```python
from build123d import *

# Parameters (mm, degrees)
F0_W     = 3.175
F0_H     = 3.175
F1_DEPTH = 6.35
F2_W     = 41.275
F2_H     = 28.575
F3_DEPTH = 6.35
F4_D     = 2.2606
F5_D     = 2.2606
F6_D     = 2.2606
F7_D     = 2.2606
F8_D     = 2.2606
F9_D     = 2.2606
F10_D    = 2.2606
F11_D    = 2.2606
F12_D    = 2.2606
F13_D    = 2.2606
F14_D    = 2.2606
F15_D    = 2.2606


with BuildPart() as f1:
    # F0 (on Top) → F1 (new body)
    with BuildSketch(Plane.XY):
        with Locations((1.5875, 1.5875)):
            Rectangle(F0_W, F0_H)
        Polygon((3.175, 3.175), (3.175, 0), (50.8, 0), (50.8, 3.175), (53.975, 3.175), (53.975, 38.1), (50.8, 38.1), (50.8, 41.275), (3.175, 41.275), (3.175, 38.1), (0, 38.1), (0, 3.175), align=None)
        with Locations((52.3875, 1.5875)):
            Rectangle(F0_W, F0_H)
        with Locations((1.5875, 39.6875)):
            Rectangle(F0_W, F0_H)
        with Locations((52.3875, 39.6875)):
            Rectangle(F0_W, F0_H)
    extrude(amount=F1_DEPTH)

    # F2 (on face) → F3 (cut, through all)
    with BuildSketch(Plane(origin=(0, 0, 0), x_dir=(1, 0, 0), z_dir=(0, 0, -1))):
        with Locations((26.9875, -20.6375)):
            Rectangle(F2_W, F2_H)
    extrude(amount=-F3_DEPTH, mode=Mode.SUBTRACT)

    # F4 (through all)
    with Locations(Plane(origin=(0, 0, 0), x_dir=(1, 0, 0), z_dir=(0, 0, -1))):
        with Locations((11.1125, -3.175)):
            Hole(F4_D / 2)

    # F5 (through all)
    with Locations(Plane(origin=(0, 0, 0), x_dir=(1, 0, 0), z_dir=(0, 0, -1))):
        with Locations((21.43125, -3.175)):
            Hole(F5_D / 2)

    # F6 (through all)
    with Locations(Plane(origin=(0, 0, 0), x_dir=(1, 0, 0), z_dir=(0, 0, -1))):
        with Locations((32.54375, -3.175)):
            Hole(F6_D / 2)

    # F7 (through all)
    with Locations(Plane(origin=(0, 0, 0), x_dir=(1, 0, 0), z_dir=(0, 0, -1))):
        with Locations((42.8625, -3.175)):
            Hole(F7_D / 2)

    # F8 (through all)
    with Locations(Plane(origin=(0, 0, 0), x_dir=(1, 0, 0), z_dir=(0, 0, -1))):
        with Locations((11.1125, -38.1)):
            Hole(F8_D / 2)

    # F9 (through all)
    with Locations(Plane(origin=(0, 0, 0), x_dir=(1, 0, 0), z_dir=(0, 0, -1))):
        with Locations((21.43125, -38.1)):
            Hole(F9_D / 2)

    # F10 (through all)
    with Locations(Plane(origin=(0, 0, 0), x_dir=(1, 0, 0), z_dir=(0, 0, -1))):
        with Locations((32.54375, -38.1)):
            Hole(F10_D / 2)

    # F11 (through all)
    with Locations(Plane(origin=(0, 0, 0), x_dir=(1, 0, 0), z_dir=(0, 0, -1))):
        with Locations((42.8625, -38.1)):
            Hole(F11_D / 2)

    # F12 (through all)
    with Locations(Plane(origin=(0, 0, 0), x_dir=(1, 0, 0), z_dir=(0, 0, -1))):
        with Locations((3.175, -9.525)):
            Hole(F12_D / 2)

    # F13 (through all)
    with Locations(Plane(origin=(0, 0, 0), x_dir=(1, 0, 0), z_dir=(0, 0, -1))):
        with Locations((3.175, -31.75)):
            Hole(F13_D / 2)

    # F14 (through all)
    with Locations(Plane(origin=(0, 0, 0), x_dir=(1, 0, 0), z_dir=(0, 0, -1))):
        with Locations((50.8, -9.525)):
            Hole(F14_D / 2)

    # F15 (through all)
    with Locations(Plane(origin=(0, 0, 0), x_dir=(1, 0, 0), z_dir=(0, 0, -1))):
        with Locations((50.8, -31.75)):
            Hole(F15_D / 2)


solid = f1.part
```
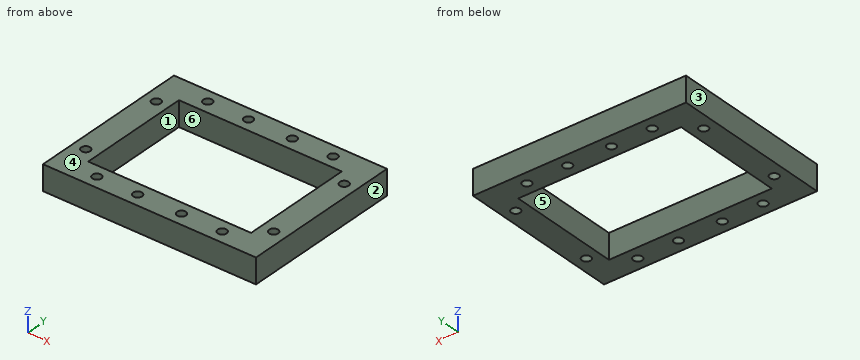
Can you work these out from the model? Positions are in its coordinate system, mm. Face numbers are marked on the shaded views. A direction names the side the tool comes from. Coordinates: 2 decimals unless noted, no trailing zeros. Loops run counter-clockwise (first coordinate to the right, second up) from the corner with the lowest first, then second, coordinate; pieces in that order, holes last. Notation, with made-up numbers: (16.25, 45.25) - (47.25, 45.25) arc R19 ccw to (47.25, 56.25) - close; hole circle Ø10 at (75, 77). An arc over 180 degrees is marked (long way). Use a Markdown table: item, result.
Item 1: We'd pull the mould along X, two halves only. Please class the marked faces 3, 4, 5 and 6: released by +X, released by -X, zero draft, split by the parting line, or undercut.
Numbers:
| item | result |
|---|---|
| face 3 | released by -X |
| face 4 | zero draft |
| face 5 | undercut |
| face 6 | undercut |
Item 2: Will this pin go through, and if not, where does the flat tip stop? pin 1 (1.4 mm diameter, centred on x = 42.86, y = 3.18, fed in from +Z).
Numbers:
| item | result |
|---|---|
| pin 1 | passes through |
Item 3: I want a section at D-D on x = 50.8. Please give me the cut outline in (y, z) (3 decimals).
Numbers:
| item | result |
|---|---|
| outline | (0, 0) - (8.395, 0) - (8.395, 6.35) - (0, 6.35) - close; (10.655, 0) - (30.62, 0) - (30.62, 6.35) - (10.655, 6.35) - close; (32.88, 0) - (41.275, 0) - (41.275, 6.35) - (32.88, 6.35) - close |
Item 4: I want a section at C-C on y = 16. Please give me the cut outline in (x, z) (3 decimals).
Numbers:
| item | result |
|---|---|
| outline | (0, 0) - (6.35, 0) - (6.35, 6.35) - (0, 6.35) - close; (47.625, 0) - (53.975, 0) - (53.975, 6.35) - (47.625, 6.35) - close |
Item 5: For the marked faces 1 and 2, which set-ups out of +Z, -Z, +X, -X, +Y, -Y let a thin tool reach every point of the face, with its end or its side?
Numbers:
| item | result |
|---|---|
| face 1 | +Z, -Z |
| face 2 | +Z, -Z, +X, +Y, -Y |
Item 6: I want a section at A-A on x = 23.5. Please give me the cut outline in (y, z) (3 decimals), and give its area (3 significant figures).
Numbers:
| item | result |
|---|---|
| outline | (0, 0) - (6.35, 0) - (6.35, 6.35) - (0, 6.35) - close; (34.925, 0) - (41.275, 0) - (41.275, 6.35) - (34.925, 6.35) - close |
| area | 80.6 mm2 |
Item 7: I want a section at B-B on y = 31.75. Please give me the cut outline in (x, z) (3 decimals).
Numbers:
| item | result |
|---|---|
| outline | (0, 0) - (2.045, 0) - (2.045, 6.35) - (0, 6.35) - close; (4.305, 0) - (6.35, 0) - (6.35, 6.35) - (4.305, 6.35) - close; (47.625, 0) - (49.67, 0) - (49.67, 6.35) - (47.625, 6.35) - close; (51.93, 0) - (53.975, 0) - (53.975, 6.35) - (51.93, 6.35) - close |
Item 8: If I drill on probe 1 along X at (y, z) = (38.1, 3) (3 decimals); probe 2 along X at (y, z) = (22, 0.5) (3 decimals); probe 3 along Y at (x, z) = (14, 3.5) (3 decimals), over which ranges is the centre line in solid material (lowest first)? Write a range as from..to.
Numbers:
| item | result |
|---|---|
| probe 1 | x = 0..9.982, 12.243..20.301, 22.562..31.413, 33.674..41.732, 43.993..53.975 |
| probe 2 | x = 0..6.35, 47.625..53.975 |
| probe 3 | y = 0..6.35, 34.925..41.275 |
